Build history of the part. All positions in model axes, mm. Face numbers are marked on the shaded views. A direction names the side the tool comes from. Round coordinates to 2 decimals unless told otherwise and drop trailing zeros. Write each loop counter-clockwise with the first axis right and the second up, starting at its lowest first coordinate (ties: lowest second). Pieces come first, ordered by that corner, then holes. Notation, with made-up numbers: (82, -6) -> (111, -6) arc R17 cw to (111, 20) -> close; hole circle Ø6 at (44, -27). An arc over 180 degrees is marked (long way). Return JSON: item names as keys, results as strings.
Autodesk Inventor part; units mm, degrees
ref_plane "YZ Plane" through (0, 0, 0) normal (1, 0, 0) x (0, 1, 0)
ref_plane "XZ Plane" through (0, 0, 0) normal (0, 1, 0) x (-1, 0, 0)
ref_plane "XY Plane" through (0, 0, 0) normal (0, 0, 1) x (1, 0, 0)
sketch "Esquisse1" plane through (0, 0, 0) normal (0, 1, 0) x (-1, 0, 0)
  circle A0 centre (0, 0) radius 6
  dimension "d0" = 12
extrude "Extrusion1" add sketch "Esquisse1" along normal blind 1
sketch "Esquisse2" plane through (0, 1, 0) normal (0, 1, 0) x (1, 0, 0)
  circle A0 centre (0, 0) radius 6
  circle A1 centre (0, 0) radius 3
  dimension "d3" = 6
extrude "Extrusion2" add sketch "Esquisse2" along normal blind 100 contours A1
fillet "Congé1" radius 2 1 edges at (6, 0, 0)
properties part number "mat"
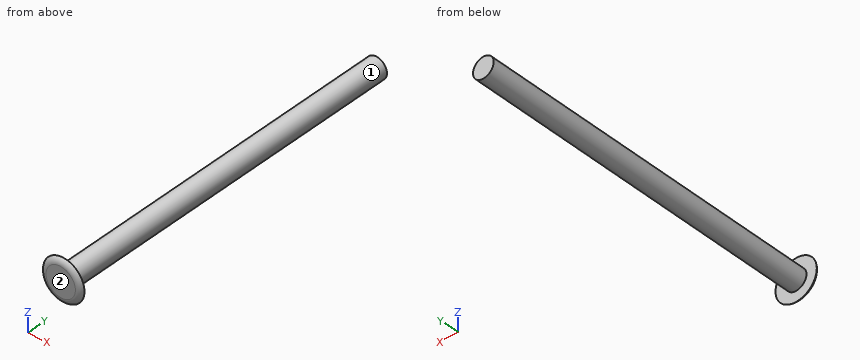
Q1. 3-axis set-ups, long thin cutter, end or side, ignore diameter. For the marked faces 1 and 2: which of +Z, -Z, +X, -X, +Y, -Y reach the whole face in a straight line?
Verdict:
{"face 1": "+Y", "face 2": "+Z, -Z, +X, -X, -Y"}
Q2. Saw through at C-C on y = 26.5. List the corners of the cut face in (x, z).
Verdict:
{"outline": "circle Ø6 at (0, 0)"}
Q3. Pin check, flat tips, straight feed: pin 1 Ø3 at (y, z) = (51.5, 2) entering from +X; pin 2 Ø3 at (x, y) = (1, 85) entering from -Z; pin 3 Ø1.5 at (y, z) = (42, 2) entering from -X. Stop position of each tip, or through.
Verdict:
{"pin 1": "stops at x = 2.96", "pin 2": "stops at z = -3", "pin 3": "stops at x = -2.73"}
Q4. Saw through at A-A on z = 0. List the corners of the cut face in (x, y).
Verdict:
{"outline": "(-6, 1) arc R2 ccw to (-4.27, 0) -> (4.27, 0) arc R2 ccw to (6, 1) -> (3, 1) -> (3, 101) -> (-3, 101) -> (-3, 1) -> close"}
Q5. Saw through at B-B on x = 0. List the corners of the cut face in (y, z), then the cut area to 3 significant figures.
Verdict:
{"outline": "(0, -4.27) arc R2 ccw to (1, -6) -> (1, -3) -> (101, -3) -> (101, 3) -> (1, 3) -> (1, 6) arc R2 ccw to (0, 4.27) -> close", "area": "611 mm²"}
Q6. Wall check: L1, parallel to X at y = 43, z = 0; L2, parallel to Y at x = 2.5, z = 2.5; L3, parallel to Z at x = -0.25, y = 24.5. Give the ranges that are in metal, low to high.
Verdict:
{"L1": "x = -3 to 3", "L2": "y = 0 to 1", "L3": "z = -2.99 to 2.99"}
